Design review of the part built by this model. Coordinates are the model's own, in mm. A direction names the side the tool comes from. Round coordinates to 2 decimals unless told otherwise and drop trailing zeros. Loops run counter-clockwise (first coordinate to the right, second up) from the corner with the lowest first, then second, coordinate; pieces in that order, holes last. Notation, with made-up numbers: M 66.25,73.5 L 83.25,73.5 A21 ccw 83.25,101.5 Z; hole C -3,58.5 d1. An arc over 180 degrees is marked long. One line per item, written item: value. Start each with the question number.
Item 1: For faces 1 (the flat face through (-37.65, 92.51, 2.54)), 2 (the flat face through (-39.27, 95.17, 2.54)), 3 (the flat face through (39.589, 100.944, 2.539)), 4 (the flat face through (35.893, 89.465, 2.539)), list the 3-axis set-ups (+Z, -Z, +X, -X, +Y, -Y) from which the entire face can be reached by the end or side of a thin tool; tool diameter is ignored.
Item 2: Clearance check with flat-ended pins moving along their axes: pin 1 (12 mm diameter, centred on x = 15.5, y = 106, fed in from -Z); pin 2 (1 mm diameter, centred on x = -6, z = 4, fed in from +Y); pin 3 (1.5 mm diameter, centred on y = 96, z = 2, fed in from +X). State where each tip first meets the part, or that it passes through.
Item 3: We need section D-D (y = 104.25). Write out the cut boundary in (x, z).
Item 4: Mouldability with a two-part tool opening along X and no side actions: class faces 5 (the flat face through (-32.89, 89.34, 2.54)), 6 (the flat face through (-1, 99, 5.15)), 7 (the cylindrical face through (0.6, 110.1, 2.5)) as released by +X, released by -X, zero draft, split by the parting line, or undercut.
Item 5: For line 1 along Y through (x, z) = (0.5, 3.55); line 2 along Y through (x, z) = (37.5, 0.4); line 3 along X through (y, z) = (92.75, 4.05), list the stretches that pass through material, from the lowest coordinate up.
Item 6: We need section B-B (y = 90). Write out the cut boundary in (x, z), then the cut area to 3 significant figures.
Item 7: We need section C-C (x = -13). Write out the cut boundary in (y, z).
Item 8: We need section A-A (z = 3.2). Write out the cut boundary in (x, y).
from build123d import *

# Parameters (mm, degrees)
BOSS_EXTRUDE1_DEPTH = 5.15


with BuildPart() as part:
    # Sketch1 → Boss-Extrude1 (new body)
    with BuildSketch(Plane.XY):
        with BuildLine():
            Line((-32.057735027, 87.9), (32.057735027, 87.9))
            Line((32.057735027, 87.9), (33.694332379, 90.734669766))
            Line((33.694332379, 90.734669766), (38.154363209, 88.159669766))
            Line((38.154363209, 88.159669766), (39.912093048, 91.204147153))
            Line((39.912093048, 91.204147153), (35.452062218, 93.779147153))
            Line((35.452062218, 93.779147153), (37.009792057, 96.477214379))
            Line((37.009792057, 96.477214379), (41.469822887, 93.902214379))
            Line((41.469822887, 93.902214379), (43.227552726, 96.946691766))
            Line((43.227552726, 96.946691766), (38.767521896, 99.521691766))
            Line((38.767521896, 99.521691766), (40.433263841, 102.406841447))
            ThreePointArc((40.433263841, 102.406841447), (0, 110.1), (-40.433263841, 102.406841447))
            Line((-40.433263841, 102.406841447), (-38.767521896, 99.521691766))
            Line((-38.767521896, 99.521691766), (-43.227552726, 96.946691766))
            Line((-43.227552726, 96.946691766), (-41.469822887, 93.902214379))
            Line((-41.469822887, 93.902214379), (-37.009792057, 96.477214379))
            Line((-37.009792057, 96.477214379), (-35.452062218, 93.779147153))
            Line((-35.452062218, 93.779147153), (-39.912093048, 91.204147153))
            Line((-39.912093048, 91.204147153), (-38.154363209, 88.159669766))
            Line((-38.154363209, 88.159669766), (-33.694332379, 90.734669766))
            Line((-33.694332379, 90.734669766), (-32.057735027, 87.9))
        make_face()
    extrude(amount=BOSS_EXTRUDE1_DEPTH)


solid = part.part
A:
1. face 1: +Z, -Z, -X
1. face 2: +Z, -Z
1. face 3: +Z, -Z, +X
1. face 4: +Z, -Z, -Y
2. pin 1: z = 0
2. pin 2: y = 109.96
2. pin 3: x = 43.11
3. outline: M -35.41,0 L 35.41,0 L 35.41,5.15 L -35.41,5.15 Z
4. face 5: undercut
4. face 6: zero draft
4. face 7: split by the parting line
5. line 1: 87.9 to 110.1
5. line 2: 88.54 to 92.6, 96.19 to 103.52
5. line 3: -37.23 to 37.23
6. outline: M -39.22,0 L -34.97,0 L -34.97,5.15 L -39.22,5.15 Z; M -33.27,0 L 33.27,0 L 33.27,5.15 L -33.27,5.15 Z; M 34.97,0 L 39.22,0 L 39.22,5.15 L 34.97,5.15 Z
6. area: 386 mm2
7. outline: M 87.9,0 L 109.33,0 L 109.33,5.15 L 87.9,5.15 Z
8. outline: M -43.23,96.95 L -41.47,93.9 L -37.01,96.48 L -35.45,93.78 L -39.91,91.2 L -38.15,88.16 L -33.69,90.73 L -32.06,87.9 L 32.06,87.9 L 33.69,90.73 L 38.15,88.16 L 39.91,91.2 L 35.45,93.78 L 37.01,96.48 L 41.47,93.9 L 43.23,96.95 L 38.77,99.52 L 40.43,102.41 A110.1 ccw -40.43,102.41 L -38.77,99.52 Z
